Autodesk Inventor part; units mm, degrees
ref_plane "YZ Plane" through (0, 0, 0) normal (1, 0, 0) x (0, 1, 0)
ref_plane "XZ Plane" through (0, 0, 0) normal (0, 1, 0) x (-1, 0, 0)
ref_plane "XY Plane" through (0, 0, 0) normal (0, 0, 1) x (1, 0, 0)
sketch "スケッチ1" plane through (0, 0, 0) normal (0, 0, 1) x (1, 0, 0)
  line L0 (-40, 5) -> (40, 5)
  line L1 (40, 5) -> (40, 0)
  line L2 (40, 0) -> (-40, 0)
  line L3 (-40, 0) -> (-40, 5)
  point P0 (0, 0)
  dimension "d5" = 40
  dimension "d6" = 80
  dimension "d7" = 5
  dimension "d8" = 0
extrude "押し出し1" add sketch "スケッチ1" along normal blind 80
sketch "スケッチ5" plane through (-40, 0, 0) normal (0, -1, 0) x (1, 0, 0)
  circle A0 centre (40, 40) radius 25
  point P0 (40, 0)
  dimension "d19" = 50
extrude "押し出し4" add sketch "スケッチ5" along normal blind 15
sketch "スケッチ6" plane through (0, -15, 40) normal (0, -1, 0) x (1, 0, 0)
  circle A0 centre (0, 0) radius 25
  circle A1 centre (0, 0) radius 2.5
  point P0 (0, -40)
  dimension "d22" = 5
extrude "押し出し5" cut sketch "スケッチ6" against normal blind 20 contours A1
sketch "スケッチ10" plane through (-40, 0, 0) normal (0, -1, 0) x (1, 0, 0)
  line L0 (80, 0) -> (0, 0)
  line L1 (80, 0) -> (80, 80)
  line L2 (0, 80) -> (5.2, 80)
  line L3 (5.2, 80) -> (5.2, 0)
  line L4 (5.2, 0) -> (0, 0)
  line L5 (0, 0) -> (0, 80)
  line L6 (80, 80) -> (74.8, 80)
  line L7 (74.8, 80) -> (74.8, 0)
  line L8 (74.8, 0) -> (80, 0)
  line L9 (80, 0) -> (80, 80)
  point P0 (40, 0)
  dimension "d70" = 5.2
  dimension "d71" = 5.2
extrude "押し出し9" cut sketch "スケッチ10" against normal blind 2.2
sketch "スケッチ11" plane through (-40, 2.2, 0) normal (0, -1, 0) x (1, 0, 0)
  line L0 (5.2, 0) -> (5.2, 80)
  line L1 (0, 80) -> (5.2, 80)
  line L2 (5.2, 80) -> (5.2, 69.9)
  line L3 (5.2, 69.9) -> (0, 69.9)
  line L4 (0, 69.9) -> (0, 80)
  line L5 (0, 0) -> (5.2, 0)
  line L6 (5.2, 0) -> (5.2, 10.1)
  line L7 (5.2, 10.1) -> (0, 10.1)
  line L8 (0, 10.1) -> (0, 0)
  point P0 (40, 0)
  dimension "d76" = 10.1
  dimension "d77" = 10.1
extrude "押し出し10" cut sketch "スケッチ11" against normal through all
sketch "スケッチ12" plane through (-40, 2.2, 0) normal (0, -1, 0) x (1, 0, 0)
  line L0 (74.8, 80) -> (74.8, 0)
  line L1 (74.8, 80) -> (80, 80)
  line L2 (80, 80) -> (74.8, 80)
  line L3 (74.8, 80) -> (74.8, 69.9)
  line L4 (74.8, 69.9) -> (80, 69.9)
  line L5 (80, 69.9) -> (80, 80)
  line L6 (80, 0) -> (74.8, 0)
  line L7 (74.8, 0) -> (74.8, 10.1)
  line L8 (74.8, 10.1) -> (80, 10.1)
  line L9 (80, 10.1) -> (80, 0)
  point P0 (40, 0)
  dimension "d80" = 10.1
  dimension "d81" = 10.1
extrude "押し出し11" cut sketch "スケッチ12" against normal through all
sketch "スケッチ13" plane through (-34.8, 5, 0) normal (0, 1, 0) x (1, 0, 0)
  line L0 (74.8, -10.1) -> (69.6, -10.1)
  line L1 (0, 0) -> (0, -10.1)
  line L2 (0, -10.1) -> (-5.2, -10.1)
  line L3 (-5.2, -69.9) -> (0, -69.9)
  line L4 (69.6, -80) -> (69.6, -69.9)
  line L5 (69.6, -69.9) -> (74.8, -69.9)
  point P0 (34.8, 0)
  point P1 (-2, -10.1)
  point P2 (-2, -69.9)
  point P3 (71.6, -69.9)
  point P4 (71.6, -10.1)
  dimension "d84" = 2
  dimension "d85" = 2
  dimension "d86" = 2
  dimension "d87" = 2
hole "Hole2" at (-36.8, 5, 10.1) at (-36.8, 5, 69.9) at (36.8, 5, 69.9) at (36.8, 5, 10.1) direction (0, -1, 0) diameter 4 end through all
sketch "スケッチ14" plane through (0, -15, 40) normal (0, -1, 0) x (1, 0, 0)
  circle A0 centre (0, 0) radius 2.5
  line L0 (-2.5, 16) -> (2.5, 16)
  line L1 (2.5, 16) -> (2.5, 6)
  line L2 (2.5, 6) -> (-2.5, 6)
  line L3 (-2.5, 6) -> (-2.5, 16)
  point P0 (0, -40)
  dimension "d95" = 5
  dimension "d96" = 6
  dimension "d97" = 10
extrude "押し出し12" cut sketch "スケッチ14" against normal through all contours L0 L1 L2 L3
fillet "フィレット6" radius 2 4 edges at (-2.5, -5, 56) (2.5, -5, 56) (2.5, -5, 46) (-2.5, -5, 46)
sketch "スケッチ16" plane through (0, -15, 40) normal (0, -1, 0) x (1, 0, 0)
  line L0 (-2.5, 8) -> (-2.5, 14)
  line L1 (2.5, 14) -> (2.5, 8)
  line L2 (0.5, 6) -> (-0.5, 6)
  circle A0 centre (0, 0) radius 2.5
  circle A1 centre (0, 0) radius 25
  arc A2 (-7.5, 18.5405) -> (7.5, 18.5405) centre (0, 0) ccw
  line L3 (-7.5, 18.5405) -> (-7.5, -7.5)
  line L4 (-7.5, -7.5) -> (7.5, -7.5)
  line L5 (7.5, -7.5) -> (7.5, 18.5405)
  arc A3 (7.5, 18.5405) -> (-7.5, 18.5405) centre (0, 0) ccw
  point P0 (0, -40)
  dimension "d104" = 40
  dimension "d105" = 5
  dimension "d106" = 5
  dimension "d107" = 7.5
extrude "押し出し14" cut sketch "スケッチ16" against normal up to surface (15 mm away) contours L3 L4 L5 A2
fillet "フィレット7" radius 7.5 2 edges at (7.5, -7.5, 32.5) (-7.5, -7.5, 32.5)
fillet "フィレット8" radius 2 2 edges at (7.5, -7.5, 58.5405) (-7.5, -7.5, 58.5405)
sketch "スケッチ17" plane through (0, -15, 40) normal (0, -1, 0) x (1, 0, 0)
  line L0 (0.5, 6) -> (-0.5, 6)
  circle A0 centre (0, 0) radius 2.5
  circle A1 centre (0, 0) radius 22.5
  line L1 (0, 0) -> (0, 22.5)
  line L2 (0, 0) -> (19.4856, -11.25)
  line L3 (0, 0) -> (-19.4856, -11.25)
  point P0 (0, -40)
  point P1 (19.4856, -11.25)
  dimension "d112" = 45
  dimension "d113" = 120
  dimension "d114" = 120
hole "Hole3" at (0, -15, 62.5) at (19.4856, -15, 28.75) at (-19.4856, -15, 28.75) direction (0, 1, 0) diameter 2.459 end through all
equation "\"d9\" = d6"
equation "\"d77\" = d76"
equation "\"d81\" = d80"
properties part number "JointB0" material "ポリエチレン、低密度"
Read the model definition and answer for the solid it produces. Units are mm, in the model's axes. A direction names the side the tool comes from. Give positions to 0.01 mm unless a question says otherwise; leave off trailing zeros. Write each loop counter-clockwise with the first axis right and the second up, starting at its lowest first coordinate (ties: lowest second). Pieces come first, ordered by that corner, then holes. Notation, with made-up numbers: (61.25, 66) - (69.25, 66) arc R22 cw to (69.25, 84) - close; hole circle Ø9 at (86.5, 71.5). An arc over 180 degrees is marked (long way). Return JSON: item names as keys, results as strings.
Q1. Given P1, Ø5.5, axis at x = -36, z = 55, coming from the -Y side; P2, Ø1.1, axis at x = 0, y = -6, coming from the -Z side; P3, Ø10, axis at x = 17.5, y = -6, coming from the +Z side, each flat-ended and moving along its own axis, determine where each tip first touches the part or whether it passes through.
Reply:
{"P1": "y = 0", "P2": "z = 15", "P3": "z = 61.65"}
Q2. A cutting plane is placed at D-D, the plane x = 22. Determine the outline of the cut face in (y, z).
Reply:
{"outline": "(-15, 28.13) - (0, 28.13) - (0, 0) - (5, 0) - (5, 80) - (0, 80) - (0, 51.87) - (-15, 51.87) - close"}
Q3. Consider line 1 along Z through (x, y) = (0, -4); line 2 along X through (y, z) = (-7, 41); line 3 along X through (y, z) = (-1, 28.75). Determine where each line is inside the solid, lowest interval first. Write a range as [from, to].
Reply:
{"line 1": "[15, 20], [32.5, 37.5], [42.5, 46], [56, 61.27], [63.73, 65]", "line 2": "[-24.98, -19.97], [-7.5, -2.29], [2.29, 7.5], [19.97, 24.98]", "line 3": "[-22.33, -20.72], [-18.26, -16.54], [16.54, 18.26], [20.72, 22.33]"}
Q4. A cutting plane is placed at B-B, the plane y = -11.5. Count the separate pieces of the cut face and the enclosed holes in it, and give its area (3 significant figures).
Reply:
{"separate pieces": "1", "enclosed holes": "6", "area": "1,010 mm²"}
Q5. For faces 5 (the face through (-2.5, -5, 51)), 6 (the face through (-8.55, -7.4, 57.05)), 7 (the face through (37, 2.2, 40)), determine the directions among +Z, -Z, +X, -X, +Y, -Y from which every point of the face is accessible in a straight line to the end or side of a thin tool.
Reply:
{"face 5": "+Y, -Y", "face 6": "-Y", "face 7": "+Z, -Z, +X, -Y"}
Q6. A cutting plane is placed at C-C, the plane z = 28.75. Determine the outline of the cut face in (x, y).
Reply:
{"outline": "(-40, 2.2) - (-34.8, 2.2) - (-34.8, 0) - (-22.33, 0) - (-22.33, -15) - (-20.72, -15) - (-20.72, 5) - (-40, 5) - close; (-18.26, -15) - (-16.54, -15) - (-16.54, 0) - (16.54, 0) - (16.54, -15) - (18.26, -15) - (18.26, 5) - (-18.26, 5) - close; (20.72, -15) - (22.33, -15) - (22.33, 0) - (34.8, 0) - (34.8, 2.2) - (40, 2.2) - (40, 5) - (20.72, 5) - close"}
Q7. A cutting plane is placed at A-A, the plane z = 62.5. Determine the outline of the cut face in (x, y).
Reply:
{"outline": "(-40, 2.2) - (-34.8, 2.2) - (-34.8, 0) - (-10.9, 0) - (-10.9, -15) - (-1.23, -15) - (-1.23, 5) - (-40, 5) - close; (1.23, -15) - (10.9, -15) - (10.9, 0) - (34.8, 0) - (34.8, 2.2) - (40, 2.2) - (40, 5) - (1.23, 5) - close"}
Q8. For a pull along X with two mould halves and no side action, classify faces 1 (the face through (-40, 4, 40)), 2 (the face through (1.9, -4.86, 55.43)), 3 (the face through (40, 4, 40)), 4 (the face through (-5.42, -7.395, 64.406)) as released by +X, released by -X, zero draft, split by the parting line, or undercut.
Reply:
{"face 1": "released by -X", "face 2": "undercut", "face 3": "released by +X", "face 4": "split by the parting line"}
